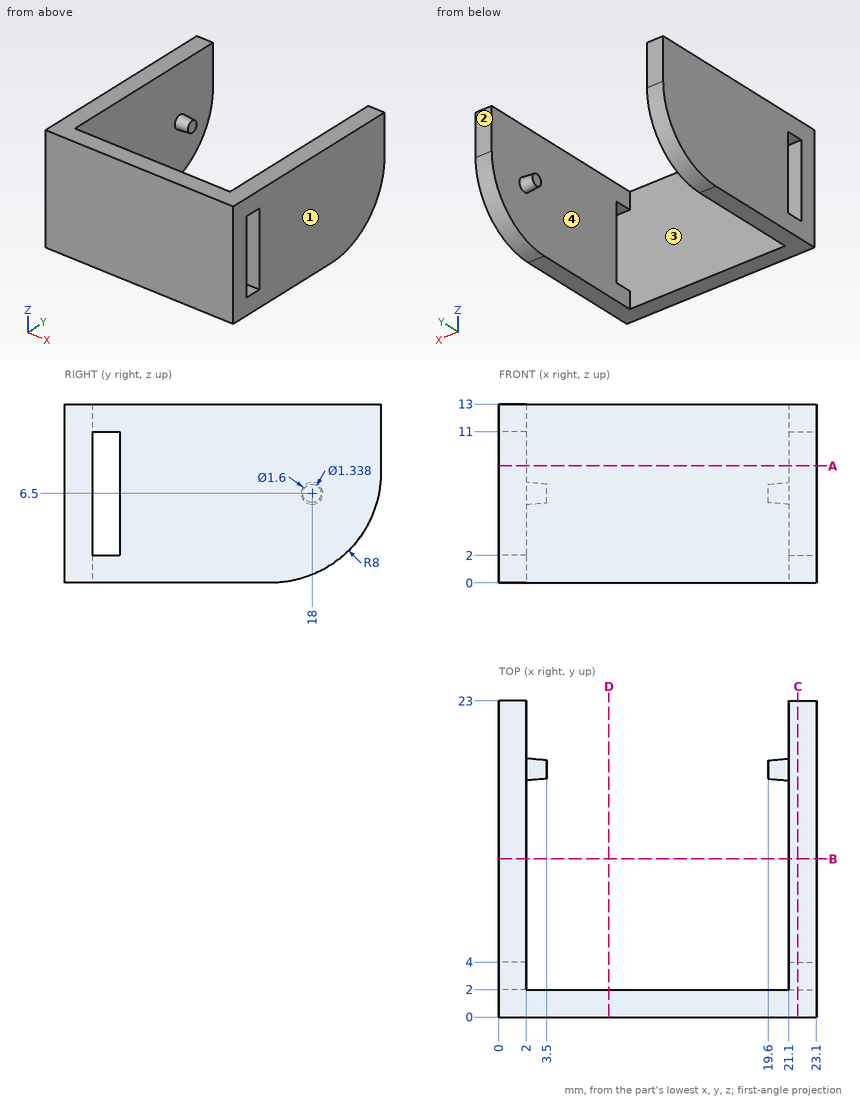
Part print with two shaded views. Sizes in mm from the minimum x, y, z corner. Round coordinates to 2 decimals unless told otherwise and drop trailing zeros. Order: outer loops, then holes, each group sorted by start corner. A loop starts at its lowest first (then second) coordinate and runs counter-clockwise, first axis right, second up.
(1) Band-saw the part on B-B (y = 11.5). List the corners of the cut face in (x, z).
(2) Band-saw the part on A-A (z = 8.5). List the corners of the cut face in (x, y), then the cut area to 3 significant figures.
(3) Band-saw the part on D-D (x = 8). List the corners of the cut face in (y, z).
(4) Band-saw the part on C-C (x = 21.75). List the corners of the cut face in (y, z).
(5) Drill centre lines: line 1 (X direction, y = 5.75, z = 8); line 2 (Y direction, x = 6.25, z = 6.5); line 3 (Y direction, x = 21.5, z = 6.5). Where is each one in solid material? Low to high.
(6) Pull direction X, two halves, no side cores. Call the marked faces 1, 2, 3 and 4: released by +X, released by -X, zero draft, split by the parting line, or undercut.
(7) Pin check, flat tip, straight feed: pin 1 (6.5 mm diameter, centred on x = 13.5, z = 5, fed in from +Y). Stop position of the tip, or through.
Verdict:
1. outline: (0, 0) - (2, 0) - (2, 13) - (0, 13) - close; (21.1, 0) - (23.1, 0) - (23.1, 13) - (21.1, 13) - close
2. outline: (0, 0) - (23.1, 0) - (23.1, 2) - (0, 2) - close; (0, 4) - (2, 4) - (2, 23) - (0, 23) - close; (21.1, 4) - (23.1, 4) - (23.1, 23) - (21.1, 23) - close
2. area: 122 mm2
3. outline: (0, 0) - (2, 0) - (2, 13) - (0, 13) - close
4. outline: (0, 0) - (15, 0) arc R8 ccw to (23, 8) - (23, 13) - (0, 13) - close; hole (2, 2) - (4, 2) - (4, 11) - (2, 11) - close
5. line 1: x = 0 to 2, 21.1 to 23.1
5. line 2: y = 0 to 2
5. line 3: y = 0 to 2, 4 to 22.86
6. face 1: released by +X
6. face 2: zero draft
6. face 3: undercut
6. face 4: undercut
7. pin 1: stops at y = 2
